Build history of the part. All positions in model axes, mm. Face numbers are marked on the shaded views. A direction names the side the tool comes from. Round coordinates to 2 decimals unless told otherwise and drop trailing zeros. Write each loop counter-clockwise with the first axis right and the second up, starting at its lowest first coordinate (ties: lowest second). Pieces come first, ordered by that corner, then holes.
Item 1: Drop flat-ended pins along their axis: pin 1 Ø2 at (x, y) = (11, -2) entering from +Z; pin 2 Ø8 at (x, z) = (0, 23.5) entering from -Y; pin 3 Ø2 at (x, y) = (-9.5, 2.5) entering from +Z. Give the stop position or say it passes through.
Item 2: Band-saw the part on B-B, the plane z = 0. Count the separate pieces of the cut face and the enclosed holes in it, then the cut area to 3 significant figures.
Item 3: Band-saw the part on C-C, the plane z = 26. Write the cut outline in (x, y), then the cut area to 3 significant figures.
Item 4: Band-saw the part on D-D, the plane y = 1.5. Write the cut outline in (x, z).
Item 5: Band-saw the part on A-A, the plane x = 0. Write the cut outline in (y, z), then the cut area to 3 significant figures.
Item 6: 3-axis set-ups, long thin cutter, end or side, ignore diameter. For the marked faces 4, 5, 6, 7 and 8: which of +Z, -Z, +X, -X, +Y, -Y reach the whole face in a straight line?
Item 7: Wall check: probe 1 along Z at (x, y) = (13, 2.35); probe 2 along X at (y, z) = (2.3, 23.5); probe 3 along Y at (x, z) = (9.5, -3.5). Give the ranges that are in metal, low to high.
Item 8: Mould opens along X. For the marked faces 1, 2 and 3 say: +X half, -X half, draft (parallel to the pull), parting line (faces both ways), or undercut.
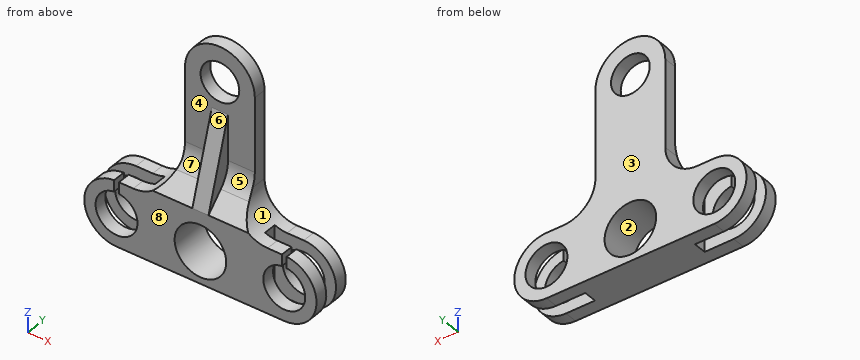
```python
from build123d import *

# Parameters (mm, degrees)
F0_R     = 3.25
F0_R_2   = 4
F0_R_3   = 3
F1_DEPTH = 3
F3_DEPTH = 12.5
F5_DEPTH = 1.25
F6_W     = 9.5
F6_H     = 2
F7_DEPTH = 12.5
F8_W     = 0.75
F8_H     = 4
F9_DEPTH = 2


# Not quite as in the source:
# - a pattern or mirror of a feature is missing from the dataset's text; its kind, count and spacing are read off the source's solid


with BuildPart() as f1:
    # F0 (on Front) → F1 (new body, symmetric)
    with BuildSketch(Plane.XZ):
        with BuildLine():
            Line((-13, -5), (13, -5))
            ThreePointArc((13, -5), (18, 0), (13, 5))
            Line((13, 5), (10.4125417955, 5))
            ThreePointArc((10.4125417955, 5), (6.8770078896, 6.4644660941), (5.4125417955, 10))
            Line((5.4125417955, 10), (5.4125417955, 6))
            Line((5.4125417955, 6), (-5.4125417955, 6))
            Line((-5.4125417955, 6), (-5.4125417955, 10))
            ThreePointArc((-5.4125417955, 10), (-6.8770078896, 6.4644660941), (-10.4125417955, 5))
            Line((-10.4125417955, 5), (-13, 5))
            ThreePointArc((-13, 5), (-18, 0), (-13, -5))
        make_face()
        with Locations((-13, 0)):
            Circle(F0_R, mode=Mode.SUBTRACT)
        Circle(F0_R_2, mode=Mode.SUBTRACT)
        with Locations((13, 0)):
            Circle(F0_R, mode=Mode.SUBTRACT)
        with BuildLine():
            Line((5.4125417955, 6), (5.4125417955, 10))
            Line((5.4125417955, 10), (5.4125417955, 23.5))
            ThreePointArc((5.4125417955, 23.5), (0, 28.9125417955), (-5.4125417955, 23.5))
            Line((-5.4125417955, 23.5), (-5.4125417955, 10))
            Line((-5.4125417955, 10), (-5.4125417955, 6))
            Line((-5.4125417955, 6), (5.4125417955, 6))
        make_face()
        with Locations((0, 23.5)):
            Circle(F0_R_3, mode=Mode.SUBTRACT)
    extrude(amount=F1_DEPTH, both=True)

    # F2 (on Right) → F3 (cut, symmetric)
    with BuildSketch(Plane.YZ):
        with BuildLine():
            Line((1, 28.9125417955), (-3, 28.9125417955))
            Line((-3, 28.9125417955), (-3, 23.5))
            Line((-3, 23.5), (-3, 10))
            Line((-3, 10), (-3, 6))
            Line((-3, 6), (-0.4644660941, 8.5355339059))
            ThreePointArc((-0.4644660941, 8.5355339059), (0.6193976626, 10.15765065), (1, 12.0710678119))
            Line((1, 12.0710678119), (1, 28.9125417955))
        make_face()
    extrude(amount=F3_DEPTH, both=True, mode=Mode.SUBTRACT)

    # F4 (on Right) → F5 (join, symmetric)
    with BuildSketch(Plane.YZ):
        Polygon((1, 19.0834104739), (-3, 6), (1.3459398516, 6), (1.3459398516, 20.2149287434), align=None)
    extrude(amount=F5_DEPTH, both=True)

    # F6 (on Top) → F7 (cut, symmetric)
    with BuildSketch(Plane.XY):
        with Locations((13.25, 0)):
            Rectangle(F6_W, F6_H)
    f7 = extrude(amount=F7_DEPTH, both=True, mode=Mode.SUBTRACT)

    # F7_copies: F7 across plane
    add(f7.mirror(Plane(origin=(0, 0, 0), x_dir=(0, 0, -1), z_dir=(-1, 0, 0))), mode=Mode.SUBTRACT)

    # F8 (on face) → F9 (cut)
    with BuildSketch(Plane.XZ.offset(3)):
        with Locations((13, 5)):
            Rectangle(F8_W, F8_H)
    f9 = extrude(amount=-F9_DEPTH, mode=Mode.SUBTRACT)

    # F9_copies: F9 across plane
    add(f9.mirror(Plane(origin=(0, 0, 0), x_dir=(0, 0, -1), z_dir=(-1, 0, 0))), mode=Mode.SUBTRACT)


solid = f1.part
```
Results:
1. pin 1: stops at z = 5.02
1. pin 2: stops at y = 1
1. pin 3: stops at z = 5.38
2. separate pieces: 6
2. enclosed holes: 0
2. area: 78.0 mm2
3. outline: (-4.8, 1) - (-1.66, 1) - (-1.66, 3) - (-4.8, 3) - close; (1.66, 1) - (4.8, 1) - (4.8, 3) - (1.66, 3) - close
3. area: 12.6 mm2
4. outline: (-13, -5) - (13, -5) arc R5 ccw to (13, 5) - (10.41, 5) arc R5 cw to (5.41, 10) - (5.41, 23.5) arc R5.41 ccw to (-5.41, 23.5) - (-5.41, 10) arc R5 cw to (-10.41, 5) - (-13, 5) arc R5 ccw to start; hole circle Ø6.5 at (-13, 0); hole circle Ø8 at (0, 0); hole circle Ø6 at (0, 23.5); hole circle Ø6.5 at (13, 0)
5. outline: (-3, -5) - (3, -5) - (3, -4) - (-3, -4) - close; (-3, 4) - (3, 4) - (3, 20.5) - (1, 20.5) - (1, 19.08) - (-3, 6) - close; (1, 26.5) - (3, 26.5) - (3, 28.91) - (1, 28.91) - close
5. area: 78.0 mm2
6. face 4: +Z, -Y
6. face 5: +Z, +X, -Y
6. face 6: +Z, +X, -X, -Y
6. face 7: +Z, -X, -Y
6. face 8: +Z, -Z, +X, -X, -Y
7. probe 1: z = -5 to -3.25, 3.25 to 5
7. probe 2: x = -5.41 to -3, 3 to 5.41
7. probe 3: y = -3 to -1, 1 to 3
8. face 1: +X half
8. face 2: undercut
8. face 3: draft
